Geometry: final body of the model. Coordinates: model frame, mm. A direction names the side the tool comes from. Round coordinates to 2 decimals unless told otherwise and drop trailing zeros. Loops run counter-clockwise (first coordinate to the right, second up) from the corner with the lowest first, then second, coordinate; pieces in that order, holes last. Notation, with made-up numbers: M 78.25,-7.5 L 98.25,-7.5 A27 ccw 98.25,26.5 Z; hole C 57.5,49.25 d1. An arc over 180 degrees is marked long. Return JSON: item names as keys, results as strings.
from build123d import *

# Parameters (mm, degrees)
SKETCH_1_R          = 7.5
SKETCH_1_R_2        = 2.55
EXTRUDE_1_DEPTH     = 5.8
SKETCH_2_W          = 20
SKETCH_2_H          = 20
SKETCH_2_R          = 2.55
EXTRUDE_2_DEPTH     = 5.8
FILLET_1_R          = 5
SKETCH_3_OUTSIDE_W  = 130.308
SKETCH_3_OUTSIDE_H  = 130.308
CUT_EXTRUDE_1_DEPTH = 95.517934806


with BuildPart() as part:
    # ｽｹｯﾁ1 → ﾎﾞｽ - 押し出し1 (new body)
    with BuildSketch(Plane.XY):
        with BuildLine():
            Line((-50, -60), (50, -60))
            Line((50, -60), (50, -30))
            ThreePointArc((50, -30), (0, 20), (-50, -30))
            Line((-50, -30), (-50, -60))
        make_face()
        Circle(SKETCH_1_R, mode=Mode.SUBTRACT)
        with Locations((-40, -50)):
            Circle(SKETCH_1_R_2, mode=Mode.SUBTRACT)
        with Locations((0, -50)):
            Circle(SKETCH_1_R_2, mode=Mode.SUBTRACT)
        with Locations((40, -50)):
            Circle(SKETCH_1_R_2, mode=Mode.SUBTRACT)
    extrude(amount=EXTRUDE_1_DEPTH)

    # ｽｹｯﾁ2 → ﾎﾞｽ - 押し出し2 (add)
    # profile 1 of 2: a face of its own
    with BuildSketch(Plane.XY.offset(5.8)):
        with Locations((-40, -70)):
            Rectangle(SKETCH_2_W, SKETCH_2_H)
        with Locations((-40, -70)):
            Circle(SKETCH_2_R, mode=Mode.SUBTRACT)
    # profile 2 of 2: a face of its own
    with BuildSketch(Plane.XY.offset(5.8)):
        with Locations((40, -70)):
            Rectangle(SKETCH_2_W, SKETCH_2_H)
        with Locations(Location((40, -70, 0), (0, 0, 180))):
            Circle(SKETCH_2_R, mode=Mode.SUBTRACT)
    extrude(amount=-EXTRUDE_2_DEPTH)

    # ﾌｨﾚｯﾄ1
    fillet_1_edges = [part.edges().sort_by_distance(p)[0] for p in [
        (-50, -80, 2.9),
        (-30, -60, 2.9),
        (-30, -80, 2.9),
        (30, -60, 2.9),
        (50, -80, 2.9),
        (30, -80, 2.9),
    ]]
    fillet(fillet_1_edges, radius=FILLET_1_R)

    # ｽｹｯﾁ3 outside → ｶｯﾄ - 押し出し1 (cut, through all)
    with BuildSketch(Plane(origin=(0, 0, 0), x_dir=(-1, 0, 0), z_dir=(0, 0, -1))):
        with Locations((0, -30)):
            Rectangle(SKETCH_3_OUTSIDE_W, SKETCH_3_OUTSIDE_H)
        with BuildLine():
            Line((-45.734623444, -32.014236411), (-23.619608507, -16.533725955))
            ThreePointArc((-23.619608507, -16.533725955), (-15.994862618, -13.854068569), (-8.086439492, -15.519648718))
            ThreePointArc((-8.086439492, -15.519648718), (0, -17.5), (8.086439492, -15.519648718))
            ThreePointArc((8.086439492, -15.519648718), (15.994862618, -13.854068569), (23.619608507, -16.533725955))
            Line((23.619608507, -16.533725955), (45.734623444, -32.014236411))
            ThreePointArc((45.734623444, -32.014236411), (48.869786763, -35.588451808), (50, -40.206555616))
            Line((50, -40.206555616), (50, -75))
            ThreePointArc((50, -75), (48.535533906, -78.535533906), (45, -80))
            Line((45, -80), (35, -80))
            ThreePointArc((35, -80), (31.464466094, -78.535533906), (30, -75))
            Line((30, -75), (30, -65))
            ThreePointArc((30, -65), (28.535533906, -61.464466094), (25, -60))
            Line((25, -60), (-25, -60))
            ThreePointArc((-25, -60), (-28.535533906, -61.464466094), (-30, -65))
            Line((-30, -65), (-30, -75))
            ThreePointArc((-30, -75), (-31.464466094, -78.535533906), (-35, -80))
            Line((-35, -80), (-45, -80))
            ThreePointArc((-45, -80), (-48.535533906, -78.535533906), (-50, -75))
            Line((-50, -75), (-50, -40.206555616))
            ThreePointArc((-50, -40.206555616), (-48.869786763, -35.588451808), (-45.734623444, -32.014236411))
        make_face(mode=Mode.SUBTRACT)
    extrude(amount=-CUT_EXTRUDE_1_DEPTH, mode=Mode.SUBTRACT)


solid = part.part
Q1. Pull-direction query (X, two-part tool) for faces 3 (the cylindrical face through (48.9, -35.65, 2.86)), 4 (the flat face through (40, -80, 3)), 5 (the flat face through (30, -70, 3)); classes: pulls with the +X half, pulls with the -X half, needs draft (parallel to the pull), parting line crosses it, or undercut.
Determined:
{"face 3": "pulls with the +X half", "face 4": "needs draft", "face 5": "undercut"}
Q2. Reachability of faces 1 (the cylindrical face through (29, -62, 3)), 2 (the cylindrical face through (-42.548, -49.888, 2.859)) from +Z, -Z, +X, -X, +Y, -Y: full face, straight path, thin tool, end or side. Return the list, or none.
Determined:
{"face 1": "+Z, -Z, -Y", "face 2": "+Z, -Z"}
Q3. Section query A-A (z = 1). Output: boundary loops of the cut face in (x, y), plus the area to 3 significant figures.
Determined:
{"outline": "M -50,-75 A5 ccw -45,-80 L -35,-80 A5 ccw -30,-75 L -30,-65 A5 cw -25,-60 L 25,-60 A5 cw 30,-65 L 30,-75 A5 ccw 35,-80 L 45,-80 A5 ccw 50,-75 L 50,-40.21 A10 ccw 45.73,-32.01 L 23.62,-16.53 A15 ccw 8.09,-15.52 A17.5 cw -8.09,-15.52 A15 ccw -23.62,-16.53 L -45.73,-32.01 A10 ccw -50,-40.21 Z; hole C -40,-70 d5.1; hole C -40,-50 d5.1; hole C 0,-50 d5.1; hole C 40,-70 d5.1; hole C 40,-50 d5.1", "area": "4,590 mm^2"}
Q4. Section query B-B (x = -40). Output: boundary loops of the cut face in (y, z).
Determined:
{"outline": "M -80,0 L -72.55,0 L -72.55,5.8 L -80,5.8 Z; M -67.45,0 L -52.55,0 L -52.55,5.8 L -67.45,5.8 Z; M -47.45,0 L -28,0 L -28,5.8 L -47.45,5.8 Z"}
Q5. Material intervals for L1, parallel to Y at x = -40, z = 2.65; L2, parallel to X at y = -67, z = 2.35; L3, parallel to X at y = -50.5, z = 4.6, sorted ascending.
Determined:
{"L1": "y = -80 to -72.55, -67.45 to -52.55, -47.45 to -28", "L2": "x = -50 to -30, 30 to 50", "L3": "x = -50 to -42.5, -37.5 to -2.5, 2.5 to 37.5, 42.5 to 50"}
Q6. Section query D-D (x = 0). Output: boundary loops of the cut face in (y, z).
Determined:
{"outline": "M -60,0 L -52.55,0 L -52.55,5.8 L -60,5.8 Z; M -47.45,0 L -17.5,0 L -17.5,5.8 L -47.45,5.8 Z"}
Q7. Pin query (flat end, axial travel): pin 1 (2 mm diameter, centred on x = -36.5, z = 2.5, fed in from +Y); pin 2 (2 mm diameter, centred on y = -30, z = 3.5, fed in from +X); pin 3 (1 mm diameter, centred on x = 15.5, z = 2.5, fed in from -Y); pin 4 (3 mm diameter, centred on x = -40, y = -70, fed in from +Z). Return the tip coordinate at first contact, or that it passes through.
Determined:
{"pin 1": "stops at y = -24.85", "pin 2": "stops at x = 44.29", "pin 3": "stops at y = -60", "pin 4": "passes through"}
Q8. Section query C-C (y = -70). Output: boundary loops of the cut face in (x, z).
Determined:
{"outline": "M -50,0 L -42.55,0 L -42.55,5.8 L -50,5.8 Z; M -37.45,0 L -30,0 L -30,5.8 L -37.45,5.8 Z; M 30,0 L 37.45,0 L 37.45,5.8 L 30,5.8 Z; M 42.55,0 L 50,0 L 50,5.8 L 42.55,5.8 Z"}
